from build123d import *

# Parameters (mm, degrees)
EXTRUDE_2_DEPTH      = 12
EXTRUDE_2_DEPTH_BACK = 12
SKETCH_1_R           = 68
FILLET_1_R           = 12
SKETCH_2_R           = 9.25
CUT_EXTRUDE_1_DEPTH  = 100.116093684
SKETCH_3_R           = 10.9
CUT_EXTRUDE_2_DEPTH  = 6.6
SKETCH_4_R           = 3.8
SKETCH_4_R_2         = 13.5
CUT_EXTRUDE_3_DEPTH  = 100.116093684
SKETCH_5_R           = 13.5
SKETCH_5_R_2         = 3.8
CUT_EXTRUDE_4_DEPTH  = 100.116093684


with BuildPart() as part:
    # 草图1 → 凸台-拉伸2 (new, two sides: drawn at the far end of the back side and taken through both)
    with BuildSketch(Plane.XY.offset(-EXTRUDE_2_DEPTH_BACK)):
        Circle(SKETCH_1_R)
    extrude(amount=EXTRUDE_2_DEPTH + EXTRUDE_2_DEPTH_BACK)

    # 圆角1
    fillet_1_edges = [part.edges().sort_by_distance(p)[0] for p in [
        (-68, 0, -12),
        (-68, 0, 12),
    ]]
    fillet(fillet_1_edges, radius=FILLET_1_R - 0.0001)  # a hair under: the kernel refuses the full size

    # 草图2 → 切除-拉伸1 (cut, through all)
    with BuildSketch(Plane(origin=(0, 0, -12), x_dir=(-1, 0, 0), z_dir=(0, 0, -1))):
        Circle(SKETCH_2_R)
    extrude(amount=-CUT_EXTRUDE_1_DEPTH, mode=Mode.SUBTRACT)

    # 草图3 → 切除-拉伸2 (cut)
    with BuildSketch(Plane(origin=(0, 0, -12), x_dir=(-1, 0, 0), z_dir=(0, 0, -1))):
        Circle(SKETCH_3_R)
    cut_extrude_2 = extrude(amount=-CUT_EXTRUDE_2_DEPTH, mode=Mode.SUBTRACT)

    # 镜向1: 切除-拉伸2 across plane
    add(cut_extrude_2.mirror(Plane.XY), mode=Mode.SUBTRACT)

    # 草图4 → 切除-拉伸3 (cut, through all)
    with BuildSketch(Plane.XY.offset(12)):
        with Locations((-18.05, 0)):
            Circle(SKETCH_4_R)
        with Locations((0, 18.05)):
            Circle(SKETCH_4_R)
        with Locations((18.05, 0)):
            Circle(SKETCH_4_R)
        with Locations((0, -18.05)):
            Circle(SKETCH_4_R)
        with Locations((-19.834345212, 19.834345212)):
            Circle(SKETCH_4_R_2)
        with Locations((19.834345212, 19.834345212)):
            Circle(SKETCH_4_R_2)
        with Locations((19.834345212, -19.834345212)):
            Circle(SKETCH_4_R_2)
        with Locations((-19.834345212, -19.834345212)):
            Circle(SKETCH_4_R_2)
    extrude(amount=-CUT_EXTRUDE_3_DEPTH, mode=Mode.SUBTRACT)

    # 草图5 → 切除-拉伸4 (cut, through all)
    with BuildSketch(Plane.XY.offset(12)):
        with Locations((-19.834345212, 19.834345212)):
            Circle(SKETCH_5_R)
        with Locations((-19.834345212, -19.834345212)):
            Circle(SKETCH_5_R)
        with Locations((-18.05, 0)):
            Circle(SKETCH_5_R_2)
        with BuildLine():
            ThreePointArc((-39.156189478, 13.899472133), (-41.548381428, 0.366743421), (-39.395447702, -13.206104662))
            ThreePointArc((-39.395447702, -13.206104662), (-37.565828535, -14.569320158), (-35.649438128, -13.331050964))
            ThreePointArc((-35.649438128, -13.331050964), (-33.259357653, -9.242884455), (-29.839682343, -5.967001238))
            ThreePointArc((-29.839682343, -5.967001238), (-26.643088536, 0.229347635), (-29.755578801, 6.468366442))
            ThreePointArc((-29.755578801, 6.468366442), (-33.114429859, 9.798428902), (-35.401059543, 13.938781679))
            ThreePointArc((-35.401059543, 13.938781679), (-37.292350318, 15.230314561), (-39.156189478, 13.899472133))
        make_face()
        with BuildLine():
            ThreePointArc((6.468366442, 29.755578801), (0.229347635, 26.643088536), (-5.967001238, 29.839682343))
            ThreePointArc((-5.967001238, 29.839682343), (-9.242884455, 33.259357653), (-13.331050964, 35.649438128))
            ThreePointArc((-13.331050964, 35.649438128), (-14.569320158, 37.565828535), (-13.206104662, 39.395447702))
            ThreePointArc((-13.206104662, 39.395447702), (0.366743421, 41.548381428), (13.899472133, 39.156189478))
            ThreePointArc((13.899472133, 39.156189478), (15.230314561, 37.292350318), (13.938781679, 35.401059543))
            ThreePointArc((13.938781679, 35.401059543), (9.798428902, 33.114429859), (6.468366442, 29.755578801))
        make_face()
        with BuildLine():
            ThreePointArc((29.755578801, -6.468366442), (26.643088536, -0.229347635), (29.839682343, 5.967001238))
            ThreePointArc((29.839682343, 5.967001238), (33.259357653, 9.242884455), (35.649438128, 13.331050964))
            ThreePointArc((35.649438128, 13.331050964), (37.565828535, 14.569320158), (39.395447702, 13.206104662))
            ThreePointArc((39.395447702, 13.206104662), (41.548381428, -0.366743421), (39.156189478, -13.899472133))
            ThreePointArc((39.156189478, -13.899472133), (37.292350318, -15.230314561), (35.401059543, -13.938781679))
            ThreePointArc((35.401059543, -13.938781679), (33.114429859, -9.798428902), (29.755578801, -6.468366442))
        make_face()
        with BuildLine():
            ThreePointArc((-6.468366442, -29.755578801), (-0.229347635, -26.643088536), (5.967001238, -29.839682343))
            ThreePointArc((5.967001238, -29.839682343), (9.242884455, -33.259357653), (13.331050964, -35.649438128))
            ThreePointArc((13.331050964, -35.649438128), (14.569320158, -37.565828535), (13.206104662, -39.395447702))
            ThreePointArc((13.206104662, -39.395447702), (-0.366743421, -41.548381428), (-13.899472133, -39.156189478))
            ThreePointArc((-13.899472133, -39.156189478), (-15.230314561, -37.292350318), (-13.938781679, -35.401059543))
            ThreePointArc((-13.938781679, -35.401059543), (-9.798428902, -33.114429859), (-6.468366442, -29.755578801))
        make_face()
    extrude(amount=-CUT_EXTRUDE_4_DEPTH, mode=Mode.SUBTRACT)


solid = part.part
Could you check a few things on this model? Use its own coordinates, in mm. A direction names the side the tool comes from. Round coordinates to 2 decimals unless told otherwise and drop trailing zeros. Put each result on its own line as item: value. Start each with the question number.
(1) I want a section at A-A, the plane z = -7. Give the number of separate pieces and of enclosed holes in the cut face, plus the area to 3 significant figures.
(2) For faces 4 (the cylindrical face through (-33.074, 9.746, 0.168)), 5 (the flat face through (5, -8, 5.4)), which set-ups out of +Z, -Z, +X, -X, +Y, -Y let a thin tool reach every point of the face, with its end or its side?
(3) Thinking about a two-plate mould opening in Y: for faces 1 (the cylindrical face through (-0.331, -26.643, 0.168)), 2 (the cylindrical face through (-26.644, 0.128, 0.168)), 3 (the flat face through (12, 1, 12)), which applies, released by +Y, released by -Y, zero draft, split by the parting line, or undercut?
(4) Will these pins go through, and if not, where does the flat tip stop? pin 1 (6 mm diameter, centred on x = 31.5, y = 54, fed in from -Z); pin 2 (16 mm diameter, centred on x = -19.83, y = -19.83, fed in from -Z); pin 3 (1.5 mm diameter, centred on x = 50.5, z = -3.5, fed in from +Y); pin 4 (4 mm diameter, centred on x = -11.5, z = -7.5, fed in from -Y).
(5) I need wall thicknesses on probe 1 along X at (y, z) = (6, 4.5); probe 2 along X at (y, z) = (13, 1.5); probe 3 along X at (y, z) = (-15, 8). Which ranges of each line are inside material? Lowest first, please.
Here are the results:
1. separate pieces: 1
1. enclosed holes: 13
1. area: 9,600 mm^2
2. face 4: +Z, -Z
2. face 5: +Z
3. face 1: undercut
3. face 2: undercut
3. face 3: zero draft
4. pin 1: stops at z = -11.47
4. pin 2: passes through
4. pin 3: stops at y = 45.65
4. pin 4: stops at y = -65.72
5. probe 1: x = -66.86 to -41.11, -29.18 to -7.04, 7.04 to 29.89, 41.11 to 66.86
5. probe 2: x = -66.65 to -39.46, -35.01 to -31.48, -8.19 to 8.19, 31.48 to 35.51, 39.46 to 66.65
5. probe 3: x = -63.19 to -32.44, -7.23 to -2.27, 2.27 to 7.23, 32.44 to 36.34, 38.2 to 63.19
